Here's how the part is built. I have some questions about the finished solid (model axes, mm). A direction names the side the tool comes from. Give positions to 0.01 mm unless a question says otherwise; leave off trailing zeros. Order: outer loops, then holes, each group sorted by start corner. A loop starts at its lowest first (then second) coordinate and runs counter-clockwise, first axis right, second up. Notation, with made-up numbers: M 61.25,64.25 L 100.25,64.25 A4 cw 100.25,69.25 Z; hole C -13.75,68.5 d10. An arc over 180 degrees is marked long. Use one line per item in the form item = value.
from build123d import *

# Parameters (mm, degrees)
F0_R     = 50.8
F1_DEPTH = 10.16
F2_R     = 46.5709
F3_DEPTH = 20.32
F4_R     = 30.48
F5_DEPTH = 20.32


# Not quite as in the source:
# - a feature names something its author has since deleted; it is built from what else it names


with BuildPart() as f1:
    # F0 (on Top) → F1 (new body)
    with BuildSketch(Plane.XY):
        Circle(F0_R)
    extrude(amount=F1_DEPTH)

    # F2 (on face) → F3 (join)
    with BuildSketch(Plane.XY.offset(10.16)):
        Circle(F2_R)
    extrude(amount=F3_DEPTH)

    # F4 (on face) → F5 (join)
    with BuildSketch(Plane.XY.offset(30.48)):
        Circle(F4_R)
    extrude(amount=F5_DEPTH)


solid = f1.part
Q1. I want a section at D-D on y = 34.5. Write out the boundary of the cut face in (x, z), then the cut area to 3 significant figures.
Found:
outline = M -37.29,0 L 37.29,0 L 37.29,10.16 L 31.28,10.16 L 31.28,30.48 L -31.28,30.48 L -31.28,10.16 L -37.29,10.16 Z
area = 2,030 mm²
Q2. I'm going to push flat-ended pins straight in: pin 1 Ø1.5 at (y, z) = (-33.5, 27) entering from +X; pin 2 Ø1.5 at (x, z) = (29, 37) entering from +Y; pin 3 Ø2 at (y, z) = (-4, 14.5) entering from -X. Where does each tip first touch, or does it pass through?
Found:
pin_1 = 33.11
pin_2 = 11.44
pin_3 = -46.47
Q3. On a 3-axis mill with a long thin cutter (end or side, diameter ignored), from which of +Z, -Z, +X, -X, +Y, -Y can I reach the whole of each face in a straight line? I mean faces 1 (the face through (-1, 1, 0)), 2 (the face through (-6.607, -29.755, 40.498)). Say none if no direction works.
Found:
face_1 = -Z, +X, -X, +Y, -Y
face_2 = +Z
Q4. I need wall thicknesses on L1, parallel to Z at x = 30, y = 29; L2, parallel to Z at x = -23.5, y = -42.5; L3, parallel to Y at x = 1, z = 43. Which ranges of each line are inside material? Lowest first, please.
Found:
L1 = 0 to 30.48
L2 = 0 to 10.16
L3 = -30.46 to 30.46
Q5. I want a section at C-C on z = 3.5. Write out the boundary of the cut face in (x, y), then the cut area to 3 significant figures.
Found:
outline = C 0,0 d101.6
area = 8,110 mm²
Q6. I want a section at A-A on y = 0. Write out the boundary of the cut face in (x, z).
Found:
outline = M -50.8,0 L 50.8,0 L 50.8,10.16 L 46.57,10.16 L 46.57,30.48 L 30.48,30.48 L 30.48,50.8 L -30.48,50.8 L -30.48,30.48 L -46.57,30.48 L -46.57,10.16 L -50.8,10.16 Z
